Here's how the part is built. I have some questions about the finished solid (model axes, mm). Coordinates: 2 decimals unless noted, no trailing zeros. Order: outer loops, then holes, each group sorted by start corner. A loop starts at its lowest first (then second) coordinate and runs counter-clockwise, first axis right, second up. Notation, with made-up numbers: (24.25, 89) - (36.25, 89) arc R5 cw to (36.25, 95) - close; hole circle Ø9 at (16.25, 2). An arc over 180 degrees is marked (long way). Answer as CSV lines item,"result". Start each with the question number.
Q1. Suppose I cut it at D-D (x = 16). Please give me the cut outline in (y, z).
Q2. For pin 1 Ø1.9 at (y, z) = (-4.5, -0.5) entering from -X, with a flat end and sliding along its axis, tell me the tip position at first contact or that it passes through.
Q3. I need wall thicknesses on line 1 (X direction, y = -5.5, z = 3.5). Which ranges of the line are inside material? Lowest first, please.
Q4. Suppose I cut it at A-A (z = 11.5). Count the separate pieces of the cut face and the enclosed holes in it, then the cut area to 3 significant figures.
Q5. Suppose I cut it at B-B (y = -4). Please give me the cut outline in (x, z).
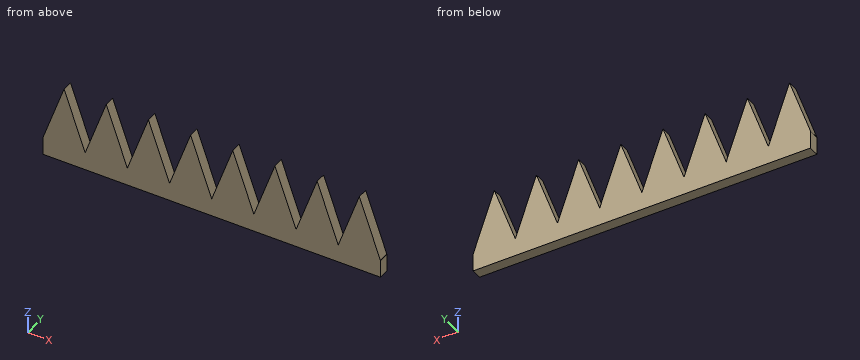
from build123d import *

# Parameters (mm, degrees)
F1_DEPTH = 6.35


with BuildPart() as f1:
    # F0 (on Front) → F1 (new body)
    with BuildSketch(Plane.XZ):
        Polygon((-101.698373, 5.38623), (-101.6, 5.38623), (-76.298373, 5.38623), (-88.998373, 41.307255), align=None)
        Polygon((-76.298373, 5.38623), (-101.6, 5.38623), (-101.6, -5.38623), (101.6, -5.38623), (101.6, 5.38623), (101.501627, 5.38623), (76.101627, 5.38623), (50.701627, 5.38623), (25.301627, 5.38623), (-0.098373, 5.38623), (-25.498373, 5.38623), (-50.898373, 5.38623), align=None)
        Polygon((-63.598373, 41.307255), (-76.298373, 5.38623), (-50.898373, 5.38623), align=None)
        Polygon((-38.198373, 41.307255), (-50.898373, 5.38623), (-25.498373, 5.38623), align=None)
        Polygon((-12.798373, 41.307255), (-25.498373, 5.38623), (-0.098373, 5.38623), align=None)
        Polygon((12.601627, 41.307255), (-0.098373, 5.38623), (25.301627, 5.38623), align=None)
        Polygon((76.101627, 5.38623), (101.501627, 5.38623), (88.801627, 41.307255), align=None)
        Polygon((38.001627, 41.307255), (25.301627, 5.38623), (50.701627, 5.38623), align=None)
        Polygon((50.701627, 5.38623), (76.101627, 5.38623), (63.401627, 41.307255), align=None)
    extrude(amount=F1_DEPTH)


solid = f1.part
Here are the results:
1,outline,"(-6.35, -5.39) - (0, -5.39) - (0, 31.7) - (-6.35, 31.7) - close"
2,pin 1,"stops at x = -101.6"
3,line 1,"x = -101.6 to 101.6"
4,separate pieces,"8"
4,enclosed holes,"0"
4,area,"1,070 mm²"
5,outline,"(-101.7, 5.39) - (-101.6, 5.39) - (-101.6, -5.39) - (101.6, -5.39) - (101.6, 5.39) - (101.5, 5.39) - (88.8, 41.31) - (76.1, 5.39) - (63.4, 41.31) - (50.7, 5.39) - (38, 41.31) - (25.3, 5.39) - (12.6, 41.31) - (-0.1, 5.39) - (-12.8, 41.31) - (-25.5, 5.39) - (-38.2, 41.31) - (-50.9, 5.39) - (-63.6, 41.31) - (-76.3, 5.39) - (-89, 41.31) - close"
